The figure shows three views and two pictorial views of one solid part (mm, origin at its lowest corner). Answer the questions. A direction names the side the tool comes from. Round coordinates to 2 decimals unless told otherwise and drop trailing zeros. Write each loop counter-clockwise with the first axis right and the second up, starting at its lowest first coordinate (ties: lowest second). Pieces come first, ordered by that corner, then holes. Notation, with made-up numbers: (41.25, 16) -> (49.25, 16) arc R17 ccw to (49.25, 32) -> close; hole circle Ø4 at (-8, -10.75). An arc over 180 degrees is marked (long way). One line per item, written item: value.
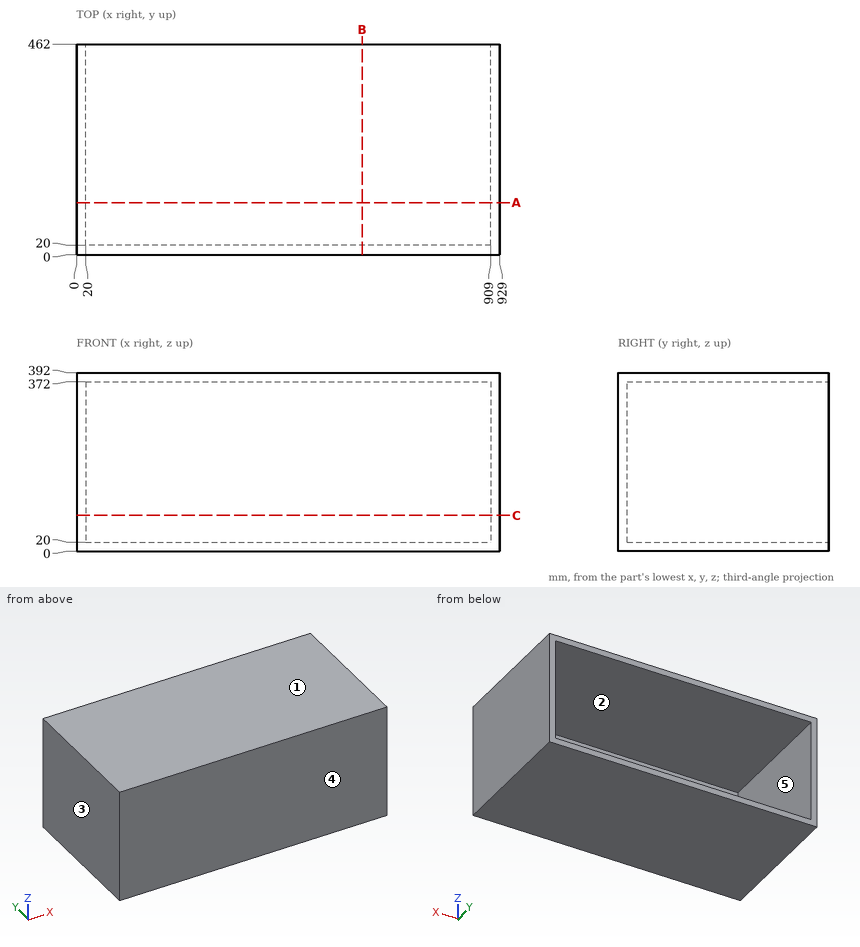
(1) Find section B-B on x = 626.5. Give the vertices of the cut face in (y, z).
Reported:
outline: (0, 0) -> (462, 0) -> (462, 20) -> (20, 20) -> (20, 372) -> (462, 372) -> (462, 392) -> (0, 392) -> close
(2) Find section A-A on y = 114. Give the vertices of the cut face in (x, z).
Reported:
outline: (0, 0) -> (929, 0) -> (929, 392) -> (0, 392) -> close; hole (20, 20) -> (909, 20) -> (909, 372) -> (20, 372) -> close
(3) A tool of negligible diameter and unlimited length cuts with its end or side. For the marked faces 4 and 5, from which of +Z, -Z, +X, -X, +Y, -Y can it reach the whole face along a straight path? Write none if from no direction.
Reported:
face 4: +Z, -Z, +X, -X, -Y
face 5: +Y
(4) Find section C-C on z = 78.5. Give the vertices of the cut face in (x, y), plus the area to 3 significant figures.
Reported:
outline: (0, 0) -> (929, 0) -> (929, 462) -> (909, 462) -> (909, 20) -> (20, 20) -> (20, 462) -> (0, 462) -> close
area: 36,300 mm2
(5) Consider probe 1 along X at (y, z) = (228, 172); probe 2 along Z at (x, y) = (101, 95); probe 3 along Y at (x, z) = (598, 80). Determine where each line is inside the solid, lowest interval first.
Reported:
probe 1: x = 0 to 20, 909 to 929
probe 2: z = 0 to 20, 372 to 392
probe 3: y = 0 to 20
(6) For a pull along Z with two mould halves and no side action, classify the marked faces 1, 2 and 3 as pulls with the +Z half, pulls with the -Z half, needs draft (parallel to the pull), parting line crosses it, or undercut.
Reported:
face 1: pulls with the +Z half
face 2: undercut
face 3: needs draft
